from build123d import *

# Parameters (mm, degrees)
SKETCH1_W                 = 300
SKETCH1_H                 = 160
BOSS_EXTRUDE1_DEPTH       = 9
SKETCH2_R                 = 14.825
SKETCH2_R_2               = 9.5
SKETCH2_R_3               = 2.75
MAIN_BUTTONS_DEPTH        = 171.238068598
SKETCH4_R                 = 1.6
SKETCH4_W                 = 9
SKETCH4_H                 = 20
LEFT_MOUNT_DEPTH          = 171.238068598
HANDLE_DEPTH              = 9
SKETCH6_W                 = 10
SKETCH6_H                 = 9
SKETCH6_W_2               = 20
CUT_EXTRUDE1_DEPTH        = 208.272767145
SKETCH7_W                 = 20
SKETCH7_H                 = 9
CUT_EXTRUDE2_DEPTH        = 208.272767145
SKETCH8_R                 = 1.6
M3_CLEARANCE_HOLES_DEPTH  = 208.272767145
MIRROR4_COPY_1_SKETCH_W   = 10
MIRROR4_COPY_1_SKETCH_H   = 9
MIRROR4_COPY_1_SKETCH_W_2 = 20
MIRROR4_COPY_1_DEPTH      = 208.272767145


with BuildPart() as part:
    # Sketch1 → Boss-Extrude1 (new body)
    with BuildSketch(Plane(origin=(0, 0, 0), x_dir=(1, 0, 0), z_dir=(0, 1, 0))):
        Rectangle(SKETCH1_W, SKETCH1_H)
    extrude(amount=BOSS_EXTRUDE1_DEPTH)

    # Sketch2 → main buttons (cut, through all)
    with BuildSketch(Plane(origin=(0, 9, 0), x_dir=(1, 0, 0), z_dir=(0, 1, 0))):
        with Locations(Location((-13, -5.325, 0), (0, 0, 270))):
            Circle(SKETCH2_R)
        with Locations(Location((20, 8.675, 0), (0, 0, 270))):
            Circle(SKETCH2_R)
        with Locations(Location((56, 2.675, 0), (0, 0, 270))):
            Circle(SKETCH2_R)
        with Locations(Location((90, -12.325, 0), (0, 0, 270))):
            Circle(SKETCH2_R)
        with Locations(Location((-72, 8.675, 0), (0, 0, 270))):
            Circle(SKETCH2_R_2)
        with Locations(Location((-94.75, 51.675, 0), (0, 0, 270))):
            Circle(SKETCH2_R_3)
        with Locations(Location((-49.25, 51.675, 0), (0, 0, 270))):
            Circle(SKETCH2_R_3)
        with Locations(Location((-94.75, -34.325, 0), (0, 0, 270))):
            Circle(SKETCH2_R_3)
        with Locations(Location((-49.25, -34.325, 0), (0, 0, 270))):
            Circle(SKETCH2_R_3)
        with Locations(Location((-6, 33.175, 0), (0, 0, 270))):
            Circle(SKETCH2_R)
        with Locations(Location((27, 47.175, 0), (0, 0, 270))):
            Circle(SKETCH2_R)
        with Locations(Location((62.5, 41.175, 0), (0, 0, 270))):
            Circle(SKETCH2_R)
        with Locations(Location((96.5, 26.175, 0), (0, 0, 270))):
            Circle(SKETCH2_R)
    extrude(amount=-MAIN_BUTTONS_DEPTH, mode=Mode.SUBTRACT)

    # Sketch4 → left mount (cut, through all)
    with BuildSketch(Plane(origin=(0, 9, 0), x_dir=(1, 0, 0), z_dir=(0, 1, 0))):
        with Locations(Location((-145.5, -26.666666667, 0), (0, 0, 270))):
            Circle(SKETCH4_R)
        with Locations(Location((-145.5, 26.666666667, 0), (0, 0, 270))):
            Circle(SKETCH4_R)
        with Locations((-145.5, 53.333333333)):
            Rectangle(SKETCH4_W, SKETCH4_H)
        with Locations((-145.5, 0)):
            Rectangle(SKETCH4_W, SKETCH4_H)
        with Locations((-145.5, -53.333333333)):
            Rectangle(SKETCH4_W, SKETCH4_H)
    left_mount = extrude(amount=-LEFT_MOUNT_DEPTH, mode=Mode.SUBTRACT)

    # Sketch3 → handle (add)
    with BuildSketch(Plane(origin=(0, 9, 0), x_dir=(1, 0, 0), z_dir=(0, 1, 0))):
        with BuildLine():
            Line((-150, -80), (-150, 80))
            Line((-150, 80), (-170.5, 80))
            ThreePointArc((-170.5, 80), (-184.995689014, 73.995689014), (-191, 59.5))
            Line((-191, 59.5), (-191, -59.5))
            ThreePointArc((-191, -59.5), (-184.995689014, -73.995689014), (-170.5, -80))
            Line((-170.5, -80), (-150, -80))
        make_face()
        with BuildLine():
            Line((-183, -59.5), (-183, 59.5))
            ThreePointArc((-183, 59.5), (-170.5, 72), (-158, 59.5))
            Line((-158, 59.5), (-158, -59.5))
            ThreePointArc((-158, -59.5), (-170.5, -72), (-183, -59.5))
        make_face(mode=Mode.SUBTRACT)
    handle = extrude(amount=-HANDLE_DEPTH)

    # Mirror1: left mount, handle across plane
    add(left_mount.mirror(Plane(origin=(0, 0, 0), x_dir=(0, 0, 1), z_dir=(1, 0, 0))), mode=Mode.SUBTRACT)
    add(handle.mirror(Plane(origin=(0, 0, 0), x_dir=(0, 0, 1), z_dir=(1, 0, 0))))

    # Sketch6 → Cut-Extrude1 (cut, through all)
    with BuildSketch(Plane(origin=(0, 9, 0), x_dir=(1, 0, 0), z_dir=(0, 1, 0))):
        with Locations((133, 72.5)):
            Rectangle(SKETCH6_W, SKETCH6_H)
        with Locations((84.666666667, 72.5)):
            Rectangle(SKETCH6_W_2, SKETCH6_H)
    cut_extrude1 = extrude(amount=-CUT_EXTRUDE1_DEPTH, mode=Mode.SUBTRACT)

    # Mirror3: Cut-Extrude1 across plane
    add(cut_extrude1.mirror(Plane(origin=(0, 0, 0), x_dir=(0, 0, 1), z_dir=(1, 0, 0))), mode=Mode.SUBTRACT)

    # Sketch7 → Cut-Extrude2 (cut, through all)
    with BuildSketch(Plane(origin=(0, 9, 0), x_dir=(1, 0, 0), z_dir=(0, 1, 0))):
        with Locations((31.333333333, 72.5)):
            Rectangle(SKETCH7_W, SKETCH7_H)
        with Locations((-31.333333333, 72.5)):
            Rectangle(SKETCH7_W, SKETCH7_H)
    cut_extrude2 = extrude(amount=-CUT_EXTRUDE2_DEPTH, mode=Mode.SUBTRACT)

    # Sketch8 → M3 clearance holes (cut, through all)
    with BuildSketch(Plane(origin=(0, 9, 0), x_dir=(1, 0, 0), z_dir=(0, 1, 0))):
        with Locations(Location((-111.333333333, 72.5, 0), (0, 0, 270))):
            Circle(SKETCH8_R)
        with Locations(Location((0, 72.5, 0), (0, 0, 270))):
            Circle(SKETCH8_R)
        with Locations(Location((111.333333333, 72.5, 0), (0, 0, 270))):
            Circle(SKETCH8_R)
    m3_clearance_holes = extrude(amount=-M3_CLEARANCE_HOLES_DEPTH, mode=Mode.SUBTRACT)

    # Mirror4: Cut-Extrude1, Cut-Extrude2, M3 clearance holes across plane
    add(cut_extrude1.mirror(Plane.XY), mode=Mode.SUBTRACT)
    add(cut_extrude2.mirror(Plane.XY), mode=Mode.SUBTRACT)
    add(m3_clearance_holes.mirror(Plane.XY), mode=Mode.SUBTRACT)

    # Mirror4 copy 1 sketch → Mirror4 copy 1 (cut, through all)
    with BuildSketch(Plane(origin=(0, 9, 0), x_dir=(-1, 0, 0), z_dir=(0, 1, 0))):
        with Locations((133, 72.5)):
            Rectangle(MIRROR4_COPY_1_SKETCH_W, MIRROR4_COPY_1_SKETCH_H)
        with Locations((84.666666667, 72.5)):
            Rectangle(MIRROR4_COPY_1_SKETCH_W_2, MIRROR4_COPY_1_SKETCH_H)
    extrude(amount=-MIRROR4_COPY_1_DEPTH, mode=Mode.SUBTRACT)


solid = part.part
Verification items for the finished model (mm, model axes). Round coordinates to 2 decimals unless told otherwise and drop trailing zeros.
1. Section check A-A on y = 1.75. State how many separate pieces and enclosed holes the cut face has, then the cut area to 3 significant figures.
Final values:
separate pieces: 1
enclosed holes: 43
area: 45,000 mm2
2. Thickness scan on L1, parallel to X at y = 3.75, z = 60; L2, parallel to Z at x = -134, y = 3; L3, parallel to Z at x = 69, y = 8. Record the ranges inside material, lowest first.
Final values:
L1: x = -190.99 to -182.99, -158.01 to -150, -141 to 141, 150 to 158.01, 182.99 to 190.99
L2: z = -80 to -77, -68 to 68, 77 to 80
L3: z = -80 to -54.5, -27.85 to -9.8, 4.45 to 80
3. Release check for a two-part mould opening along X. For faces 1 (the flat face through (31, 5, 77)), 2 (the flat face through (-2, 5, -80)), 3 (the flat face through (146, 5, 63.333)) record: +X half, -X half, draft (parallel to the pull), parting line (faces both ways), or undercut.
Final values:
face 1: undercut
face 2: draft
face 3: undercut
